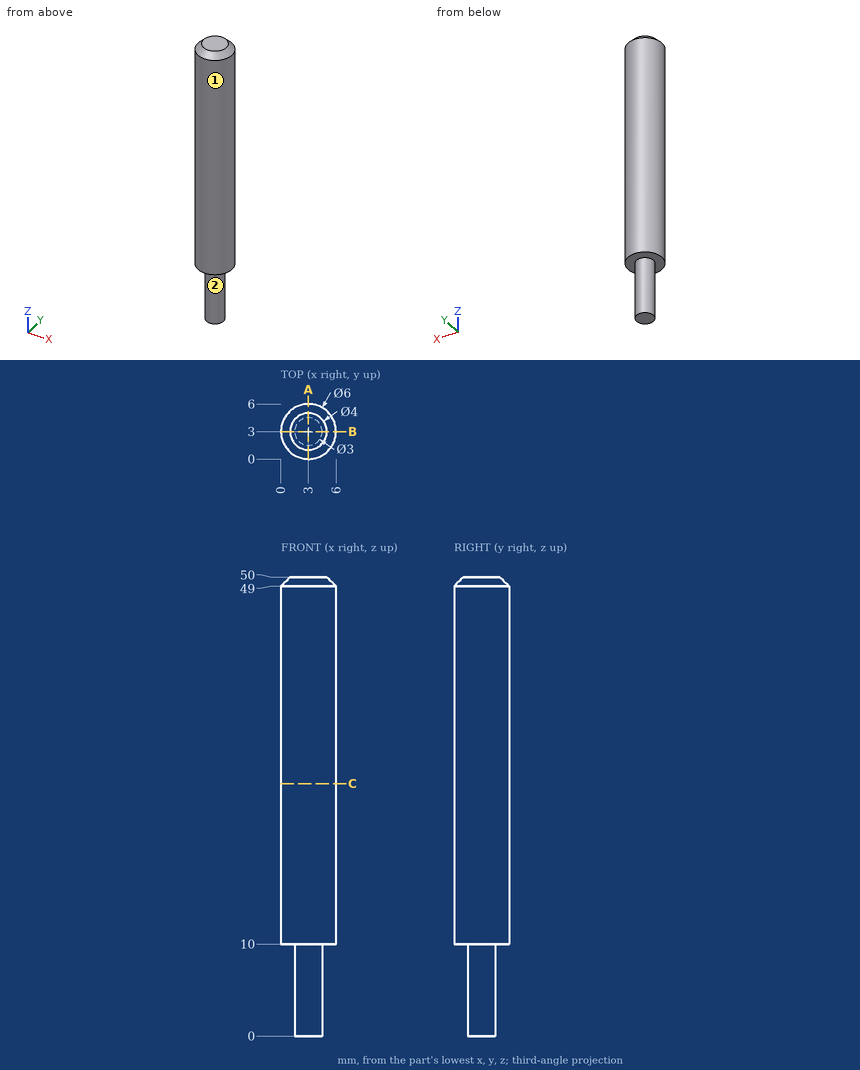
Here's the drawing with two shaded views (mm, measured from the low corner). I have some questions. A direction names the side the tool comes from. Coordinates: 2 decimals unless noted, no trailing zeros. Order: outer loops, then holes, each group sorted by start corner. A loop starts at its lowest first (then second) coordinate and runs counter-clockwise, first axis right, second up. Notation, with made-up numbers: (85.25, 18.25) - (107.25, 18.25) arc R5 ccw to (107.25, 22.25) - close; hole circle Ø8 at (11, 3). An arc over 180 degrees is marked (long way). Answer in a Markdown table with one row per item. Add a question column.
(1) I need wall thicknesses on L1, parallel to Z at x = 4.3, y = 4.05; L2, parallel to X at y = 3.1, z = 18.5; L3, parallel to Y at x = 1.7, z = 47. Which ranges of each line are inside material? Lowest first, please.
(2) If we section it at A-A, the plane x = 3: Please give me the cut outline in (y, z).
(3) If we section it at C-C, the plane z = 27.5: Please give me the cut outline in (x, y), then the cut area to 3 significant figures.
(4) On a 3-axis mill with a long thin cutter (end or side, diameter ignored), from which of +Z, -Z, +X, -X, +Y, -Y can I reach the whole of each face in a straight line? I mean the marked faces 1 and 2. Say none if no direction works.
Results are:
| question | item | result |
|---|---|---|
| 1 | L1 | z = 10 to 50 |
| 1 | L2 | x = 0 to 6 |
| 1 | L3 | y = 0.3 to 5.7 |
| 2 | outline | (0, 10) - (1.5, 10) - (1.5, 0) - (4.5, 0) - (4.5, 10) - (6, 10) - (6, 49) - (5, 50) - (1, 50) - (0, 49) - close |
| 3 | outline | circle Ø6 at (3, 3) |
| 3 | area | 28.3 mm2 |
| 4 | face 1 | +Z, -Z |
| 4 | face 2 | -Z |
